Geometry: final body of the model. Coordinates: model frame, mm. Coordinates: 2 decimals unless noted, no trailing zeros. Loops run counter-clockwise (first coordinate to the right, second up) from the corner with the lowest first, then second, coordinate; pieces in that order, holes last. Notation, with made-up numbers: (-19.5, 71) - (21.5, 71) arc R15 cw to (21.5, 86) - close; hole circle Ø6 at (-27.75, -19). An arc over 180 degrees is marked (long way). Return JSON: item names as keys, results as strings.
from build123d import *

# Parameters (mm, degrees)
SKETCH_2_W          = 85
SKETCH_2_H          = 55
EXTRUDE_3_DEPTH     = 8
SKETCH_5_W          = 80.2
SKETCH_5_H          = 50.2
CUT_EXTRUDE_1_DEPTH = 1.8
SKETCH_7_R          = 1.5
CUT_EXTRUDE_4_DEPTH = 2.2
SKETCH_8_W          = 15
SKETCH_8_H          = 10
SKETCH_8_W_2        = 10
SKETCH_8_H_2        = 15
SKETCH_8_H_3        = 12
CUT_EXTRUDE_6_DEPTH = 3


with BuildPart() as part:
    # 草图2 → 凸台-拉伸3 (new body)
    with BuildSketch(Plane(origin=(0, 0, 0), x_dir=(1, 0, 0), z_dir=(0, 1, 0))):
        with Locations((42.5, 27.5)):
            Rectangle(SKETCH_2_W, SKETCH_2_H)
    extrude(amount=EXTRUDE_3_DEPTH)

    # 草图5 → 切除-拉伸1 (cut)
    with BuildSketch(Plane(origin=(0, 8, 0), x_dir=(1, 0, 0), z_dir=(0, 1, 0))):
        with Locations((42.5, 27.5)):
            Rectangle(SKETCH_5_W, SKETCH_5_H)
    extrude(amount=-CUT_EXTRUDE_1_DEPTH, mode=Mode.SUBTRACT)

    # 草图7 → 切除-拉伸4 (cut)
    with BuildSketch(Plane(origin=(0, 6.2, 0), x_dir=(1, 0, 0), z_dir=(0, 1, 0))):
        with Locations(Location((7.4, 47.6, 0), (0, 0, 270))):
            Circle(SKETCH_7_R)
        with Locations(Location((67.6, 47.6, 0), (0, 0, 90))):
            Circle(SKETCH_7_R)
        with Locations((7.4, -2.6)):
            Circle(SKETCH_7_R)
        with Locations((67.6, -2.6)):
            Circle(SKETCH_7_R)
    extrude(amount=-CUT_EXTRUDE_4_DEPTH, mode=Mode.SUBTRACT)

    # 草图8 → 切除-拉伸6 (cut)
    with BuildSketch(Plane(origin=(0, 6.2, 0), x_dir=(1, 0, 0), z_dir=(0, 1, 0))):
        with Locations((19.9, 9.4)):
            Rectangle(SKETCH_8_W, SKETCH_8_H)
        with Locations((75.6, 35.1)):
            Rectangle(SKETCH_8_W_2, SKETCH_8_H_2)
        with Locations((34.9, 43.6)):
            Rectangle(SKETCH_8_W, SKETCH_8_H_3)
    extrude(amount=-CUT_EXTRUDE_6_DEPTH, mode=Mode.SUBTRACT)


solid = part.part
Item 1: Section query A-A, the plane x = 29. Return loops of the section in (y, z), and give its area (3 significant figures).
Worked out:
{"outline": "(0, -55) - (8, -55) - (8, -52.6) - (6.2, -52.6) - (6.2, -49.6) - (3.2, -49.6) - (3.2, -37.6) - (6.2, -37.6) - (6.2, -2.4) - (8, -2.4) - (8, 0) - (0, 0) - close", "area": "314 mm^2"}
Item 2: First-contact query: pin 1 Ø11 at (x, z) = (74.5, -35.5) entering from +Y; pin 2 Ø1.5 at (x, y) = (20, 5) entering from +Z. Flat tips, straight axial feed; report the tip coordinate or a pass-through.
Worked out:
{"pin 1": "y = 6.2", "pin 2": "z = 0"}
Item 3: Section query B-B, the plane z = -35. Return loops of the section in (x, y).
Worked out:
{"outline": "(0, 0) - (85, 0) - (85, 8) - (82.6, 8) - (82.6, 6.2) - (80.6, 6.2) - (80.6, 3.2) - (70.6, 3.2) - (70.6, 6.2) - (2.4, 6.2) - (2.4, 8) - (0, 8) - close"}
Item 4: Ray query, probe 1 along X at (y, z) = (4.7, -47.6); probe 2 along X at (y, z) = (5.25, -42.5); probe 3 along Z at (x, y) = (67.6, 5.45). Return the intervals inside material, ascending. Write a range as from..to.
Worked out:
{"probe 1": "0..5.9, 8.9..27.4, 42.4..66.1, 69.1..85", "probe 2": "0..27.4, 42.4..70.6, 80.6..85", "probe 3": "-55..-49.1, -46.1..0"}
Item 5: Section query C-C, the plane z = -47.6. Return loops of the section in (x, y), and give its area (3 significant figures).
Worked out:
{"outline": "(0, 0) - (85, 0) - (85, 8) - (82.6, 8) - (82.6, 6.2) - (69.1, 6.2) - (69.1, 4) - (66.1, 4) - (66.1, 6.2) - (42.4, 6.2) - (42.4, 3.2) - (27.4, 3.2) - (27.4, 6.2) - (8.9, 6.2) - (8.9, 4) - (5.9, 4) - (5.9, 6.2) - (2.4, 6.2) - (2.4, 8) - (0, 8) - close", "area": "477 mm^2"}
Item 6: Mould query, pull axis Z, two halves, no side actions, for faces 1 (the face through (39, 8, -1)), 2 (the face through (35, 3.2, -44)). Classes: +Z half, -Z half, draft (parallel to the pull), parting line (faces both ways), or undercut.
Worked out:
{"face 1": "draft", "face 2": "undercut"}
